Autodesk Inventor part; units mm, degrees
ref_plane "YZ Plane" through (0, 0, 0) normal (1, 0, 0) x (0, 1, 0)
ref_plane "XZ Plane" through (0, 0, 0) normal (0, 1, 0) x (-1, 0, 0)
ref_plane "XY Plane" through (0, 0, 0) normal (0, 0, 1) x (1, 0, 0)
sketch "Sketch1" plane through (0, 0, 0) normal (0, 1, 0) x (-1, 0, 0)
  line L0 (73.025, 73.025) -> (-73.025, 73.025)
  line L1 (-73.025, 73.025) -> (-73.025, -73.025)
  line L2 (-73.025, -73.025) -> (73.025, -73.025)
  line L3 (73.025, -73.025) -> (73.025, 73.025)
  line L4 (73.025, 73.025) -> (-73.025, -73.025) construction
  line L5 (-73.025, 73.025) -> (73.025, -73.025) construction
  point P0 (0, 0)
  dimension "d2" = 146.05
  dimension "d3" = 146.05
extrude "Extrusion1" add sketch "Sketch1" along normal blind 19.05
sketch "Sketch2" plane through (0, 19.05, 0) normal (0, 1, 0) x (1, 0, 0)
  circle A0 centre (0, -9.525) radius 3.175
  line L0 (73.025, 73.025) -> (-73.025, 73.025)
  line L1 (-73.025, 73.025) -> (-73.025, -73.025)
  point P0 (0, 0)
  dimension "d6" = 6.35
  dimension "d7" = 82.55
  dimension "d8" = 73.025
extrude "Extrusion2" cut sketch "Sketch2" against normal blind 19.05
sketch "Sketch3" plane through (0, 19.05, 0) normal (0, 1, 0) x (1, 0, 0)
  circle A0 centre (-63.5, -47.625) radius 4.0894
  line L0 (-73.025, 73.025) -> (-73.025, -73.025)
  line L1 (-73.025, -73.025) -> (73.025, -73.025)
  circle A1 centre (-64.6763, 28.575) radius 4.0894
  circle A2 centre (63.5, -47.625) radius 4.0894
  line L2 (73.025, -73.025) -> (73.025, 73.025)
  circle A3 centre (63.5, 28.575) radius 4.0894
  circle A4 centre (-28.575, 63.5) radius 4.0894
  line L3 (73.025, 73.025) -> (-73.025, 73.025)
  circle A5 centre (28.575, 63.5) radius 4.0894
  point P0 (0, 0)
  dimension "d11" = 8.1788
  dimension "d12" = 9.525
  dimension "d13" = 25.4
  dimension "d14" = 8.1788
  dimension "d15" = 101.6
  dimension "d16" = 8.1788
  dimension "d17" = 25.4
  dimension "d18" = 9.525
  dimension "d19" = 8.1788
  dimension "d20" = 9.525
  dimension "d21" = 101.6
  dimension "d22" = 8.1788
  dimension "d23" = 44.45
  dimension "d24" = 9.525
  dimension "d25" = 8.1788
  dimension "d26" = 101.6
extrude "Extrusion3" cut sketch "Sketch3" against normal blind 19.05 contours A0 | A1 | A2 | A3 | A4 | A5
properties part number "Part_side"
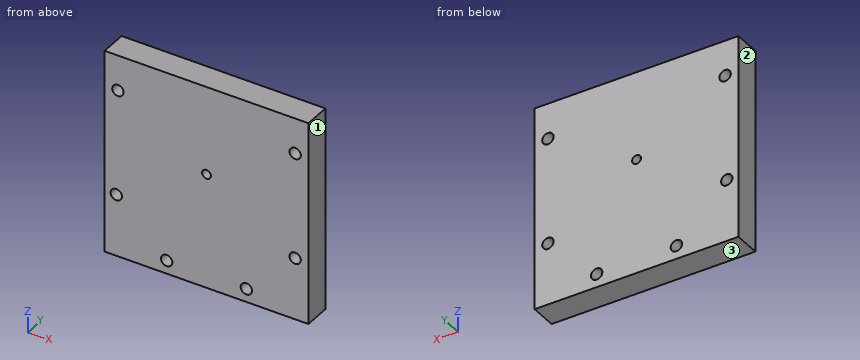
Verification items for the finished model (mm, model axes). Face numbers are marked on the shaded views. Coordinates: 2 decimals unless noted, no trailing zeros. Order: outer loops, then holes, each group sorted by start corner. A loop starts at its lowest first (then second) coordinate and runs counter-clockwise, first axis right, second up. Notation, with made-up numbers: M 88.25,43.5 L 130.25,43.5 A17 ccw 130.25,59.5 Z; hole C 17.5,35 d8. An arc over 180 degrees is marked long. One line per item, written item: value. Start each with the question number.
Item 1: Scan lines: probe 1 along X at (y, z) = (7, -63.5) (3 decimals); probe 2 along X at (y, z) = (16.75, 45.5) (3 decimals); probe 3 along Z at (x, y) = (31, 18) (3 decimals). Record each from-to range of solid material in increasing order.
Item 2: Sectioned sample at B-B (x = 0). Enter the section's corners in (y, z) (3 decimals), then the cut area to 3 significant figures.
Item 3: Sectioned sample at A-A (z = -63.5). Enter the section's corners in (x, y) (3 decimals), then the cut area to 3 significant figures.
Item 4: Sectioned sample at C-C (x = 63.5). Enter the section's corners in (y, z) (3 decimals).
Item 5: Gauge pin test, flat end, axial feed: pin 1 (7.5 mm diameter, centred on x = 28.575, z = -63.5, fed in from +Y). Record the tip position at first contact, or that the pin passes through.
Item 6: Sectioned sample at D-D (y = 5.5). Enter the section's corners in (x, z) (3 decimals), then the cut area to 3 significant figures.
Item 7: Mould release check, pull along X, two halves, no side actions. Record for the marked faces 1, 2 and 3: released by +X, released by -X, zero draft, split by the parting line, or undercut.
Conclusion:
1. probe 1: x = -73.025 to -32.664, -24.486 to 24.486, 32.664 to 73.025
1. probe 2: x = -73.025 to -66.994, -60.006 to 60.006, 66.994 to 73.025
1. probe 3: z = -73.025 to -66.793, -60.207 to 73.025
2. outline: M 0,-73.025 L 19.05,-73.025 L 19.05,6.35 L 0,6.35 Z; M 0,12.7 L 19.05,12.7 L 19.05,73.025 L 0,73.025 Z
2. area: 2,660 mm^2
3. outline: M -73.025,0 L -32.664,0 L -32.664,19.05 L -73.025,19.05 Z; M -24.486,0 L 24.486,0 L 24.486,19.05 L -24.486,19.05 Z; M 32.664,0 L 73.025,0 L 73.025,19.05 L 32.664,19.05 Z
3. area: 2,470 mm^2
4. outline: M 0,-73.025 L 19.05,-73.025 L 19.05,-32.664 L 0,-32.664 Z; M 0,-24.486 L 19.05,-24.486 L 19.05,43.536 L 0,43.536 Z; M 0,51.714 L 19.05,51.714 L 19.05,73.025 L 0,73.025 Z
5. pin 1: passes through
6. outline: M -73.025,-73.025 L 73.025,-73.025 L 73.025,73.025 L -73.025,73.025 Z; hole C -64.676,-28.575 d8.179; hole C -63.5,47.625 d8.179; hole C -28.575,-63.5 d8.179; hole C 0,9.525 d6.35; hole C 28.575,-63.5 d8.179; hole C 63.5,-28.575 d8.179; hole C 63.5,47.625 d8.179
6. area: 21,000 mm^2
7. face 1: released by +X
7. face 2: released by -X
7. face 3: zero draft
